```python
from build123d import *

# Parameters (mm, degrees)
F0_W     = 54
F0_H     = 54
F1_DEPTH = 400
F2_R     = 7
F3_DEPTH = 3


# Not quite as in the source:
# - a feature names something its author has since deleted; it is built from what else it names


with BuildPart() as f1:
    # F0 (on Front) → F1 (new body)
    with BuildSketch(Plane.XZ):
        with BuildLine():
            ThreePointArc((-28.9867345989, -60.995567819), (-30.4512006929, -57.460033913), (-33.9867345989, -55.995567819))
            Line((-33.9867345989, -55.995567819), (-83.9867345989, -55.995567819))
            ThreePointArc((-83.9867345989, -55.995567819), (-87.5222685048, -57.460033913), (-88.9867345989, -60.995567819))
            Line((-88.9867345989, -60.995567819), (-88.9867345989, -110.995567819))
            ThreePointArc((-88.9867345989, -110.995567819), (-87.5222685048, -114.5311017249), (-83.9867345989, -115.995567819))
            Line((-83.9867345989, -115.995567819), (-33.9867345989, -115.995567819))
            ThreePointArc((-33.9867345989, -115.995567819), (-30.4512006929, -114.5311017249), (-28.9867345989, -110.995567819))
            Line((-28.9867345989, -110.995567819), (-28.9867345989, -60.995567819))
        make_face()
        with Locations((-58.9867345989, -85.995567819)):
            Rectangle(F0_W, F0_H, mode=Mode.SUBTRACT)
    extrude(amount=-F1_DEPTH)

    # F2 (on face) → F3 (cut, through all)
    with BuildSketch(Plane.YZ.offset(-28.9867345989)):
        with Locations((20, -85.995567819)):
            Circle(F2_R)
        with Locations((50, -85.995567819)):
            Circle(F2_R)
        with Locations((350, -85.995567819)):
            Circle(F2_R)
        with Locations((380, -85.995567819)):
            Circle(F2_R)
    extrude(amount=-F3_DEPTH, mode=Mode.SUBTRACT)


solid = f1.part
```
Build history of the part. All positions in model axes, mm. A direction names the side the tool comes from. Round coordinates to 2 decimals unless told otherwise and drop trailing zeros. Write each loop counter-clockwise with the first axis right and the second up, starting at its lowest first coordinate (ties: lowest second). Pieces come first, ordered by that corner, then holes.
1) Band-saw the part on D-D, the plane y = 366. List the corners of the cut face in (x, z).
2) Band-saw the part on B-B, the plane y = 20. List the corners of the cut face in (x, z).
3) Drill centre lines: probe 1 along X at (y, z) = (294, -107.5); probe 2 along Z at (x, y) = (-71.5, 268.5); probe 3 along X at (y, z) = (143.5, -112). Where is each one in solid material? Low to high.
4) Band-saw the part on A-A, the plane x = -38.5. List the corners of the cut face in (y, z).
5) 3-axis set-ups, long thin cutter, end or side, ignore diameter. For faces 1 (the flat face through (-59, 197, -58.996)), 2 (the flat face through (-59, 197, -115.996)), 3 (the cylindrical face through (-30.466, 19.089, -79.055)): which of +Z, -Z, +X, -X, +Y, -Y reach the whole face in a straight line?
6) Mould opens along X. For faces 4 (the flat face through (-28.987, 197, -86)), 5 (the flat face through (-85.987, 197, -86)), 6 (the flat face through (-59, 0, -57)) say: +X half, -X half, draft (parallel to the pull), parting line (faces both ways), or undercut.
7) Band-saw the part on C-C, the plane z = -73. List the corners of the cut face in (x, y).
Ans:
1. outline: (-88.99, -111) arc R5 ccw to (-83.99, -116) - (-33.99, -116) arc R5 ccw to (-28.99, -111) - (-28.99, -61) arc R5 ccw to (-33.99, -56) - (-83.99, -56) arc R5 ccw to (-88.99, -61) - close; hole (-85.99, -113) - (-31.99, -113) - (-31.99, -59) - (-85.99, -59) - close
2. outline: (-88.99, -111) arc R5 ccw to (-83.99, -116) - (-33.99, -116) arc R5 ccw to (-28.99, -111) - (-28.99, -93) - (-31.99, -93) - (-31.99, -113) - (-85.99, -113) - (-85.99, -59) - (-31.99, -59) - (-31.99, -79) - (-28.99, -79) - (-28.99, -61) arc R5 ccw to (-33.99, -56) - (-83.99, -56) arc R5 ccw to (-88.99, -61) - close
3. probe 1: x = -88.99 to -85.99, -31.99 to -28.99
3. probe 2: z = -116 to -113, -59 to -56
3. probe 3: x = -88.88 to -85.99, -31.99 to -29.09
4. outline: (0, -116) - (400, -116) - (400, -113) - (0, -113) - close; (0, -59) - (400, -59) - (400, -56) - (0, -56) - close
5. face 1: +Y, -Y
5. face 2: -Z, +X, -X, +Y, -Y
5. face 3: +X
6. face 4: +X half
6. face 5: undercut
6. face 6: draft
7. outline: (-88.99, 0) - (-85.99, 0) - (-85.99, 400) - (-88.99, 400) - close; (-31.99, 0) - (-28.99, 0) - (-28.99, 400) - (-31.99, 400) - close
